```python
from build123d import *

# Parameters (mm, degrees)
BASE_FLANGE1_DEPTH             = 65
CHAMFER1_SIZE                  = 5
F_6_6_6_6_DIAMETER_HOLE1_D     = 6.6
F_6_6_6_6_DIAMETER_HOLE1_DEPTH = 3
F_6_6_6_6_DIAMETER_HOLE1_TIP   = 1.982840043


# Sheet-metal steps are written as plain solids
with BuildPart() as part:
    # Sketch1 → Base-Flange1 (new, symmetric)
    with BuildSketch(Plane.XY):
        with BuildLine():
            Line((-100, 0), (-53.9116, 0))
            ThreePointArc((-53.9116, 0), (-51.145681115, 1.145681115), (-50, 3.9116))
            Line((-50, 3.9116), (-50, 160))
            ThreePointArc((-50, 160), (0, 210), (50, 160))
            Line((50, 160), (50, 3.9116))
            ThreePointArc((50, 3.9116), (51.145681115, 1.145681115), (53.9116, 0))
            Line((53.9116, 0), (100, 0))
            Line((100, 0), (100, 3.175))
            Line((100, 3.175), (53.9116, 3.175))
            ThreePointArc((53.9116, 3.175), (53.390745145, 3.390745145), (53.175, 3.9116))
            Line((53.175, 3.9116), (53.175, 160))
            ThreePointArc((53.175, 160), (0, 213.175), (-53.175, 160))
            Line((-53.175, 160), (-53.175, 3.9116))
            ThreePointArc((-53.175, 3.9116), (-53.390745145, 3.390745145), (-53.9116, 3.175))
            Line((-53.9116, 3.175), (-100, 3.175))
            Line((-100, 3.175), (-100, 0))
        make_face()
    extrude(amount=BASE_FLANGE1_DEPTH, both=True)

    # Chamfer1
    chamfer1_edges = [part.edges().sort_by_distance(p)[0] for p in [
        (-100, 1.5875, -65),
        (100, 1.5875, -65),
        (-100, 1.5875, 65),
        (100, 1.5875, 65),
    ]]
    chamfer(chamfer1_edges, length=CHAMFER1_SIZE)

    # Ø6.6 (6.6) Diameter Hole1
    with Locations(Plane(origin=(75, 3.175, 0), x_dir=(0, 0, 1), z_dir=(0, 1, 0))):
        with Locations((0, 0), (0, -150)):
            Hole(F_6_6_6_6_DIAMETER_HOLE1_D / 2, depth=F_6_6_6_6_DIAMETER_HOLE1_DEPTH)
            with Locations((0, 0, -(F_6_6_6_6_DIAMETER_HOLE1_DEPTH + F_6_6_6_6_DIAMETER_HOLE1_TIP / 2))):  # 118° drill point
                Cone(0, F_6_6_6_6_DIAMETER_HOLE1_D / 2, F_6_6_6_6_DIAMETER_HOLE1_TIP, mode=Mode.SUBTRACT)


solid = part.part
```
Geometry check sheet. Reference: the model listing, model coordinates, mm. A direction names the side the tool comes from. Give positions to 0.01 mm unless a question says otherwise; leave off trailing zeros. Loops run counter-clockwise (first coordinate to the right, second up) from the corner with the lowest first, then second, coordinate; pieces in that order, holes last. Notation, with made-up numbers: M -31.5,-5 L 14.5,-5 A16 cw 14.5,12 Z; hole C -21.75,39.25 d1. An arc over 180 degrees is marked long. Write item = value, one per line.
(1) Gauge pin test, flat ends, axial feed: pin 1 Ø6 at (y, z) = (151, 10.5) entering from -X (3 decimals); pin 2 Ø23 at (x, z) = (-72.5, -13) entering from +Y (3 decimals); pin 3 Ø1.5 at (x, y) = (-53.5, 63) entering from +Z; pin 4 Ø4 at (x, z) = (21.5, -5) entering from -Y. Record the tip position at first contact, or that the pin passes through.
Answer below:
pin_1 = -53.175
pin_2 = 3.175
pin_3 = 65
pin_4 = 204.13
(2) Tool access check on faces 4 (the face through (50, 83, 1)), 5 (the face through (1.169, 213.162, 0.91)), 6 (the face through (-53.175, 83, 1)), 7 (the face through (77.783, 1.654, -1.774)), 8 (the face through (82, 3.175, 1)). Record the directions out of +Z, -Z, +X, -X, +Y, -Y that give a thin tool (end or side, any length) a straight path to the whole face; none if there is none.
Answer below:
face_4 = +Z, -Z, -Y
face_5 = +Z, -Z, +Y
face_6 = +Z, -Z, -X, +Y
face_7 = +Y
face_8 = +Z, -Z, +X, +Y
(3) Sectioned sample at A-A, the plane y = 81.5. Record the cut outline in (x, z) (3 decimals), plus the area to 4 significant figures.
Answer below:
outline = M -53.175,-65 L -50,-65 L -50,65 L -53.175,65 Z; M 50,-65 L 53.175,-65 L 53.175,65 L 50,65 Z
area = 825.5 mm2
(4) Sectioned sample at D-D, the plane z = 0. Record the cut outline in (x, y) (3 decimals), plus the area to 3 significant figures.
Answer below:
outline = M -100,0 L -78.009,0 L -78.3,0.175 L -78.3,3.175 L -100,3.175 Z; M -71.991,0 L -53.912,0 A3.912 ccw -50,3.912 L -50,160 A50 cw 50,160 L 50,3.912 A3.912 ccw 53.912,0 L 71.991,0 L 71.7,0.175 L 71.7,3.175 L 53.912,3.175 A0.737 cw 53.175,3.912 L 53.175,160 A53.175 ccw -53.175,160 L -53.175,3.912 A0.737 cw -53.912,3.175 L -71.7,3.175 L -71.7,0.175 Z; M 78.009,0 L 100,0 L 100,3.175 L 78.3,3.175 L 78.3,0.175 Z
area = 1,780 mm2
(5) Release check for a two-part mould opening along Z. For faces 1 (the face through (53.175, 81, 1)), 2 (the face through (-72.217, 1.654, -1.774)), 3 (the face through (-97, 2, 63)) record: released by +Z, released by -Z, zero draft, split by the parting line, or undercut.
Answer below:
face_1 = zero draft
face_2 = undercut
face_3 = released by +Z
(6) Sectioned sample at B-B, the plane z = -16.5. Record the cut outline in (x, y) (3 decimals).
Answer below:
outline = M -100,0 L -53.912,0 A3.912 ccw -50,3.912 L -50,160 A50 cw 50,160 L 50,3.912 A3.912 ccw 53.912,0 L 100,0 L 100,3.175 L 53.912,3.175 A0.737 cw 53.175,3.912 L 53.175,160 A53.175 ccw -53.175,160 L -53.175,3.912 A0.737 cw -53.912,3.175 L -100,3.175 Z
(7) Sectioned sample at C-C, the plane x = 75. Record the cut outline in (y, z) (3 decimals).
Answer below:
outline = M 0,-65 L 3.175,-65 L 3.175,-3.3 L 0.175,-3.3 L 0,-3.009 Z; M 0,3.009 L 0.175,3.3 L 3.175,3.3 L 3.175,65 L 0,65 Z
(8) Material ranges on line 1 (X direction, y = 122.5, z = 16) (3 decimals); line 2 (Z direction, x = -75, y = 1.55); line 3 (X direction, y = 1.3, z = 0), recorded low to high. Write a range as [from, to].
Answer below:
line_1 = [-53.175, -50], [50, 53.175]
line_2 = [-65, -3.3], [3.3, 65]
line_3 = [-100, -78.3], [-71.7, -51], [51, 71.7], [78.3, 100]
